```python
from build123d import *

# Parameters (mm, degrees)
FILLET1_R = 20


with BuildPart() as part:
    # Sketch1 → Revolve1 (revolve)
    with BuildSketch(Plane.XY):
        Polygon((0, -573.807622343), (0, -623.807622343), (250, -623.807622343), (450.694452759, 576.192377657), (400, 576.192377657), (207.667816106, -573.807622343), align=None)
    revolve(axis=Axis((0, 411.869437483, 0), (0, -1, 0)))

    # Fillet1
    fillet1_edges = [part.edges().sort_by_distance(p)[0] for p in [
        (-400, 576.192377657, 0),
        (-450.694452759, 576.192377657, 0),
        (-250, -623.807622343, 0),
    ]]
    fillet(fillet1_edges, radius=FILLET1_R)


solid = part.part
```
Verification items for the finished model (mm, model axes). Give positions to 0.01 mm unless a question says otherwise; leave off trailing zeros. Order: outer loops, then holes, each group sorted by start corner. A loop starts at its lowest first (then second) coordinate and runs counter-clockwise, first axis right, second up. Notation, with made-up numbers: M 16.25,-38.75 L 50.25,-38.75 A23 ccw 50.25,-25.75 Z; hole C 13,15.5 d5. An arc over 180 degrees is marked long. Answer in a Markdown table with one row per item. Add a question column.
Item 1: Section check B-B, the plane z = 0. Enter the section's corners in (x, y).
Item 2: Section check C-C, the plane y = 202.5. Enter the section's corners in (x, z).
Item 3: Section check D-D, the plane y = 390.5. Enter the section's corners in (x, z), and give its area (3 significant figures).
Item 4: Gauge pin test, flat ends, axial feed: pin 1 (10 mm diameter, centred on y = -58, z = -172.5, fed in from -X); pin 2 (3 mm diameter, centred on y = 166.5, z = -128, fed in from +X); pin 3 (5 mm diameter, centred on y = -430.5, z = -234, fed in from +X). Record the tip position at first contact, or that the pin passes through.
Item 5: Mould release check, pull along X, two halves, no side actions. Record for faces 1 (the flat face through (3, -623.808, 3)), 2 (the flat face through (-3, -573.808, 3)), 3 (the conical face through (-278.663, -18.987, -213.671)): released by +X, released by -X, zero draft, split by the parting line, or undercut.
Item 6: Section check A-A, the plane x = 0. Enter the section's corners in (y, z).
Item 7: Scan lines: probe 1 along Z at (x, y) = (-204, -320.5); probe 2 along X at (y, z) = (298.5, -182.5); probe 3 along Z at (x, y) = (97, 503.5). Record each from-to range of solid material in increasing order. Write a range as from..to.
Filled sheet:
| question | item | result |
|---|---|---|
| 1 | outline | M -446.8,552.89 L -252.79,-607.11 A20 ccw -233.07,-623.81 L 233.07,-623.81 A20 ccw 252.79,-607.11 L 446.8,552.89 A20 ccw 427.07,576.19 L 416.93,576.19 A20 ccw 397.21,559.49 L 207.67,-573.81 L -207.67,-573.81 L -397.21,559.49 A20 ccw -416.93,576.19 L -427.07,576.19 A20 ccw Z |
| 2 | outline | C 0,0 d776.39; hole C 0,0 d675 |
| 3 | outline | C 0,0 d839.28; hole C 0,0 d737.89 |
| 3 | area | 126,000 mm^2 |
| 4 | pin 1 | stops at x = -301.35 |
| 4 | pin 2 | stops at x = 360.7 |
| 4 | pin 3 | stops at x = 161.68 |
| 5 | face 1 | zero draft |
| 5 | face 2 | undercut |
| 5 | face 3 | split by the parting line |
| 6 | outline | M -623.81,-233.07 A20 ccw -607.11,-252.79 L 552.89,-446.8 A20 ccw 576.19,-427.07 L 576.19,-416.93 A20 ccw 559.49,-397.21 L -573.81,-207.67 L -573.81,207.67 L 559.49,397.21 A20 ccw 576.19,416.93 L 576.19,427.07 A20 ccw 552.89,446.8 L -607.11,252.79 A20 ccw -623.81,233.07 Z |
| 7 | probe 1 | z = -220.95..-144.57, 144.57..220.95 |
| 7 | probe 2 | x = -360.71..-302.81, 302.81..360.71 |
| 7 | probe 3 | z = -427.67..-375.52, 375.52..427.67 |
